Can you work these out from the drawing? Everything is in mm from the part's minimum corner. A direction names the side the tool comes from. Give positions to 0.01 mm unless a question says otherwise; leave off trailing zeros. Loops run counter-clockwise (first coordinate to the right, second up) from the corner with the lowest first, then second, coordinate; pieces in that order, holes last. Notation, with made-up numbers: (84.5, 86) - (143.5, 86) arc R18 ccw to (143.5, 104) - close; hole circle Ø6 at (78.25, -2.5). An arc over 180 degrees is marked (long way). One line per item, written item: value. Start each with the question number.
Q1. I'm going to push flat-ended pins straight in: P1, Ø3, axis at x = 49.5, y = 1.5, coming from the +Z side (3 decimals); P2, Ø2, axis at x = 78, z = 19, coming from the +Y side; P3, Ø2, axis at y = 16.5, z = 12.5, coming from the +X side. Where does each tip first touch, or does it pass through?
Q2. If I drill on line 1 (Y direction, x = 52.5, z = 10.5); line 2 (Z direction, x = 28.5, y = 4.5); line 3 (Y direction, x = 44.5, z = 30), over which ranges is the centre line in solid material (lowest first)? Write a range as from..to.
Q3. If we mould it in two halves opening along Z, with no side actions, what happens to the marked faces 3, 4 and 5? For each: released by +Z, released by -Z, zero draft, split by the parting line, or undercut.
Q4. For the marked faces 1 and 2, which set-ups out of +Z, -Z, +X, -X, +Y, -Y let a thin tool reach every point of the face, with its end or its side?
Q5. I want a section at C-C (z = 5). Please give me the cut outline in (x, y), then the cut area to 3 significant figures.
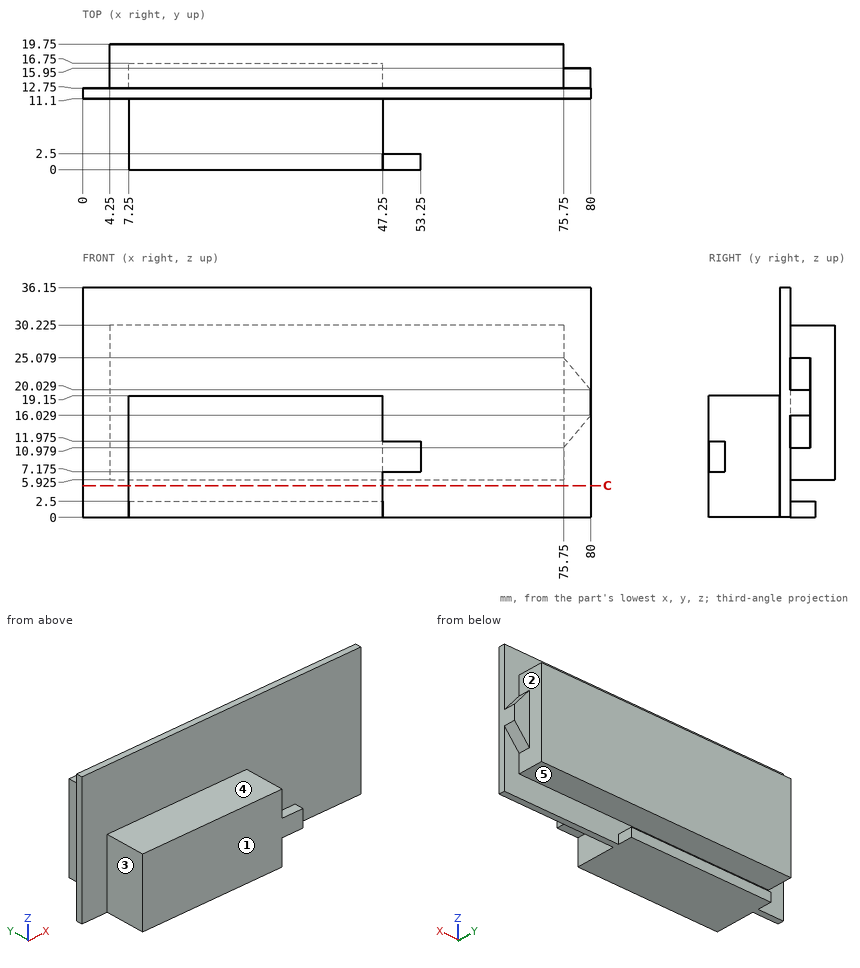
Worked answers:
1. P1: stops at z = 11.975
1. P2: stops at y = 15.95
1. P3: stops at x = 77.73
2. line 1: y = 0..2.5, 11.1..19.75
2. line 2: z = 0..19.15
2. line 3: y = 11.1..19.75
3. face 3: zero draft
3. face 4: released by +Z
3. face 5: undercut
4. face 1: +Z, -Z, +X, -X, -Y
4. face 2: +X, +Y
5. outline: (0, 11.1) - (7.25, 11.1) - (7.25, 0) - (47.25, 0) - (47.25, 11.1) - (80, 11.1) - (80, 12.75) - (0, 12.75) - close
5. area: 576 mm²
